```python
from build123d import *

# Parameters (mm, degrees)
SKETCH_R     = 1.6
PAD_DEPTH    = 3
FILLET_R     = 3
CHAMFER_SIZE = 0.2


with BuildPart() as part:
    # Sketch → Pad (new body)
    with BuildSketch(Plane.XY):
        Polygon((0, 0), (0, -20), (-42, -20), (-42, 42), (-8.5, 42), (-8.5, 32), (-16, 32), (-16, 14), (2, 14), (2, 32), (-5.5, 32), (-5.5, 42), (20, 42), (20, 0), align=None)
        with Locations((10, 32)):
            Circle(SKETCH_R, mode=Mode.SUBTRACT)
        with Locations((-32, -10)):
            Circle(SKETCH_R, mode=Mode.SUBTRACT)
    extrude(amount=PAD_DEPTH)

    # Fillet
    fillet_edges = [part.edges().sort_by_distance(p)[0] for p in [
        (-42, -20, 1.5),
        (20, 0, 1.5),
        (0, -20, 1.5),
        (-42, 42, 1.5),
        (20, 42, 1.5),
        (-5.5, 32, 1.5),
        (-5.5, 42, 1.5),
        (2, 32, 1.5),
        (-8.5, 32, 1.5),
        (-16, 32, 1.5),
        (-16, 14, 1.5),
        (2, 14, 1.5),
        (-8.5, 42, 1.5),
    ]]
    fillet(fillet_edges, radius=FILLET_R)

    # Chamfer
    chamfer_edges = [part.edges().sort_by_distance(p)[0] for p in [
        (-33.6, -10, 0),
        (8.4, 32, 0),
        (-33.6, -10, 3),
        (8.4, 32, 3),
    ]]
    chamfer(chamfer_edges, length=CHAMFER_SIZE)


solid = part.part
```
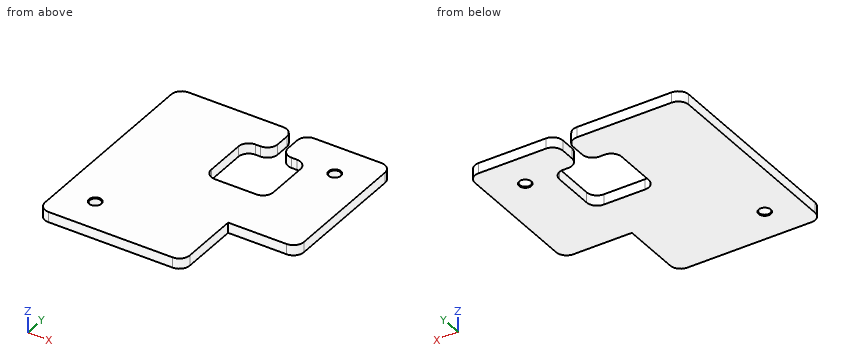
For this review, take the finished solid that the model builds, in its own axes (mm). Give positions to 0.01 mm unless a question says otherwise; leave off trailing zeros. Order: outer loops, then holes, each group sorted by start corner. A loop starts at its lowest first (then second) coordinate and runs counter-clockwise, first axis right, second up.
1) Take a section at B-B (x = -32). Give the boundary of the cut face in (y, z).
2) Take a section at A-A (y = -10). Give the boundary of the cut face in (x, z), then the cut area to 3 significant figures.
3) Wall thickness on line 1 (Y direction, x = 10, z = 1.7); line 2 (Y direction, x = -32, z = 1.55); line 3 (X direction, y = 27, z = 1.75): over which ranges is each line inside the solid? List them lowest first.
4) Take a section at D-D (y = 20). Give the boundary of the cut face in (x, z), then the cut area to 3 significant figures.
5) Insertion check: pin 1 (0.9 mm diameter, centred on x = 8.5, z = 2, fed in from -Y); pin 2 (3.5 mm diameter, centred on x = 10, y = 32, fed in from +Z); pin 3 (0.8 mm diameter, centred on x = -1.5, z = 2, fed in from -Y). Each pin has a flat end and moves straight along its axis. Give the tip position at first contact, or say it passes through.
6) Take a section at C-C (z = 1.4). State how many separate pieces and enclosed holes the cut face has, then the cut area to 3 significant figures.
Derived:
1. outline: (-20, 0) - (-11.8, 0) - (-11.6, 0.2) - (-11.6, 2.8) - (-11.8, 3) - (-20, 3) - close; (-8.4, 0.2) - (-8.2, 0) - (42, 0) - (42, 3) - (-8.2, 3) - (-8.4, 2.8) - close
2. outline: (-42, 0) - (-33.8, 0) - (-33.6, 0.2) - (-33.6, 2.8) - (-33.8, 3) - (-42, 3) - close; (-30.4, 0.2) - (-30.2, 0) - (0, 0) - (0, 3) - (-30.2, 3) - (-30.4, 2.8) - close
2. area: 116 mm2
3. line 1: y = 0 to 30.4, 33.6 to 42
3. line 2: y = -20 to -11.6, -8.4 to 42
3. line 3: x = -42 to -16, 2 to 20
4. outline: (-42, 0) - (-16, 0) - (-16, 3) - (-42, 3) - close; (2, 0) - (20, 0) - (20, 3) - (2, 3) - close
4. area: 132 mm2
5. pin 1: stops at y = 0
5. pin 2: stops at z = 2.95
5. pin 3: stops at y = -19.79
6. separate pieces: 1
6. enclosed holes: 2
6. area: 3,060 mm2
